from build123d import *

# Parameters (mm, degrees)
F0_R     = 15.5
F0_R_2   = 10.05
F1_DEPTH = 6.5
F2_DEPTH = 25.6
F3_R     = 2
F4_SIZE2 = 2
F4_SIZE  = 20
F5_SIZE  = 1


with BuildPart() as f1:
    # F0 (on Top) → F1 (new body)
    with BuildSketch(Plane.XY):
        Circle(F0_R)
        Circle(F0_R_2, mode=Mode.SUBTRACT)
        Circle(F0_R_2)
    extrude(amount=F1_DEPTH)

    # F0 (on Top) → F2 (join)
    with BuildSketch(Plane.XY):
        Circle(F0_R)
        Circle(F0_R_2, mode=Mode.SUBTRACT)
    extrude(amount=F2_DEPTH)

    # F3
    f3_edges = [f1.edges().sort_by_distance(p)[0] for p in [
        (-15.5, 0, 0),
    ]]
    fillet(f3_edges, radius=F3_R)

    # F4
    f4_edges = [f1.edges().sort_by_distance(p)[0] for p in [
        (15.5, 0, 13.8),
        (-15.5, 0, 2),
        (-15.5, 0, 25.6),
    ]]
    f4_side = f1.faces().sort_by_distance((-15.5, 0, 13.8))[0]
    chamfer(f4_edges, length=F4_SIZE, length2=F4_SIZE2, reference=f4_side)

    # F5
    f5_edges = [f1.edges().sort_by_distance(p)[0] for p in [
        (-10.05, 0, 25.6),
    ]]
    chamfer(f5_edges, length=F5_SIZE)


solid = f1.part
For this review, take the finished solid that the model builds, in its own axes (mm). A direction names the side the tool comes from. Round coordinates to 2 decimals unless told otherwise and drop trailing zeros. Order: outer loops, then holes, each group sorted by start corner. A loop starts at its lowest first (then second) coordinate and runs counter-clockwise, first axis right, second up. Notation, with made-up numbers: M -1,59.25 L 9,59.25 A32 cw 9,95.25 Z; hole C -5.5,-8 d3. An arc over 180 degrees is marked long. Use a Markdown table: item, result. Add a question column.
Item 1: Tool access review of faces 1 (the cylindrical face through (-2.018, 15.368, 3.775)), 2 (the flat face through (0, 0, 6.5)): name each direction out of +Z, -Z, +X, -X, +Y, -Y from which nothing blocks a thin tool from reaching the whole face with its end or side.
Item 2: Insertion check: pin 1 (6 mm diameter, centred on y = -12, z = 9.5, fed in from -X); pin 2 (4 mm diameter, centred on x = -6.5, z = 6, fed in from -Y); pin 3 (4 mm diameter, centred on y = -11.5, z = 19, fed in from -X). Each pin has a flat end and moves straight along its axis. Give the tip position at first contact, or say it passes through.
Item 3: Add section A-A, the plane x = 0. Give the boundary of the cut face in (y, z), then the cut area to 3 significant figures.
Item 4: Add section C-C, the plane z = 3.5. Give the boundary of the cut face in (x, y).
Item 5: Mouldability with a two-part tool opening along Y and no side actions: class faces 3 (the cylindrical face through (9.586, 3.019, 15.423)), 4 (the conical face through (13.176, -5.463, 17.962)), 5 (the flat face through (-11.1, 2.1, 25.6)) as released by +Y, released by -Y, zero draft, split by the parting line, or undercut.
Item 6: Add section D-D, the plane z = 18. Give the boundary of the cut face in (x, y), then the cut area to 3 significant figures.
Item 7: To check wall thickness, follow line 1 along Z through (x, y) = (-5, 6); line 2 along Y through (x, z) = (0, 20); line 3 along X through (y, z) = (7, 20). State the ranges of each line that lie inside material, in increasing order.
Geometry results:
| question | item | result |
|---|---|---|
| 1 | face 1 | +Z, -Z |
| 1 | face 2 | +Z |
| 2 | pin 1 | stops at x = -12.17 |
| 2 | pin 2 | stops at y = -14.82 |
| 2 | pin 3 | stops at x = -10.52 |
| 3 | outline | M -15.5,2 A2 ccw -13.5,0 L 13.5,0 A2 ccw 15.5,2 L 15.5,5.6 L 13.5,25.6 L 11.05,25.6 L 10.05,24.6 L 10.05,6.5 L -10.05,6.5 L -10.05,24.6 L -11.05,25.6 L -13.5,25.6 L -15.5,5.6 Z |
| 3 | area | 367 mm² |
| 4 | outline | C 0,0 d31 |
| 5 | face 3 | undercut |
| 5 | face 4 | split by the parting line |
| 5 | face 5 | zero draft |
| 6 | outline | C 0,0 d28.52; hole C 0,0 d20.1 |
| 6 | area | 322 mm² |
| 7 | line 1 | z = 0 to 6.5 |
| 7 | line 2 | y = -14.06 to -10.05, 10.05 to 14.06 |
| 7 | line 3 | x = -12.19 to -7.21, 7.21 to 12.19 |
